Autodesk Inventor part; units mm, degrees
ref_plane "YZ Plane" through (0, 0, 0) normal (1, 0, 0) x (0, 1, 0)
ref_plane "XZ Plane" through (0, 0, 0) normal (0, 1, 0) x (-1, 0, 0)
ref_plane "XY Plane" through (0, 0, 0) normal (0, 0, 1) x (1, 0, 0)
sketch "Sketch1" plane through (0, 0, 0) normal (0, 0, 1) x (1, 0, 0)
  line L0 (0, 0) -> (25.4, 0)
  line L1 (25.4, 0) -> (25.4, -50.8)
  line L2 (25.4, -50.8) -> (0, -50.8)
  line L3 (0, -50.8) -> (0, 0)
  line L4 (22.225, -3.175) -> (3.175, -3.175)
  line L5 (3.175, -3.175) -> (3.175, -47.625)
  line L6 (3.175, -47.625) -> (22.225, -47.625)
  line L7 (22.225, -47.625) -> (22.225, -3.175)
  dimension "d0" = 25.4
  dimension "d1" = 50.8
  dimension "d2" = 3.175
extrude "Extrusion1" add sketch "Sketch1" along normal blind 127
sketch "Sketch2" plane through (0, 0, 0) normal (0, 1, 0) x (1, 0, 0)
  circle A0 centre (12.7, -12.7) radius 11.1125
  line L0 (0, 0) -> (0, -127)
  line L1 (0, 0) -> (25.4, 0)
  circle A1 centre (12.7, -112.0904) radius 11.1125
  circle A2 centre (12.7, -211.4809) radius 11.1125
  dimension "d5" = 12.7
  dimension "d6" = 12.7
  dimension "d7" = 22.225
  dimension "d8" = 99.3904
  dimension "d9" = 99.3904
  dimension "d10" = 12.7
  dimension "d11" = 22.225
  dimension "d12" = 12.7
  dimension "d13" = 22.225
extrude "Extrusion2" cut sketch "Sketch2" against normal blind 127
sketch "Sketch3" plane through (25.4, -50.8, 0) normal (1, 0, 0) x (0, 0, -1)
  line L0 (0, 44.45) -> (-63.5, 44.45)
  line L1 (-63.5, 44.45) -> (-63.5, 6.35)
  line L2 (-63.5, 6.35) -> (0, 6.35)
  line L3 (0, 6.35) -> (0, 44.45)
  line L4 (0, 50.8) -> (-127, 50.8)
  line L5 (0, 0) -> (-127, 0)
  line L6 (0, 50.8) -> (0, 0)
  dimension "d19" = 6.35
  dimension "d20" = 6.35
  dimension "d21" = 38.1
  dimension "d22" = 63.5
  dimension "d23" = 0
extrude "Extrusion3" cut sketch "Sketch3" against normal blind 127
properties part number "C Arm"
Verification items for the finished model (mm, model axes). A direction names the side the tool comes from. Round coordinates to 2 decimals unless told otherwise and drop trailing zeros. Write each loop counter-clockwise with the first axis right and the second up, starting at its lowest first coordinate (ties: lowest second). Pieces come first, ordered by that corner, then holes.
(1) Section check D-D (z = 12.7). Enter the section's corners in (x, y), plus the area to 3 significant figures.
Returned:
outline: (0, -50.8) - (1.59, -50.8) - (1.59, -44.45) - (0, -44.45) - close; (0, -6.35) - (1.59, -6.35) - (1.59, 0) - (0, 0) - close; (23.81, -50.8) - (25.4, -50.8) - (25.4, -44.45) - (23.81, -44.45) - close; (23.81, -6.35) - (25.4, -6.35) - (25.4, 0) - (23.81, 0) - close
area: 40.3 mm2
(2) Section check C-C (x = 12.7). Enter the section's corners in (y, z) (1 decimal).
Returned:
outline: (-50.8, 0) - (-47.6, 0) - (-47.6, 1.6) - (-50.8, 1.6) - close; (-50.8, 23.8) - (-47.6, 23.8) - (-47.6, 101) - (-50.8, 101) - close; (-50.8, 123.2) - (-47.6, 123.2) - (-47.6, 127) - (-50.8, 127) - close; (-3.2, 0) - (0, 0) - (0, 1.6) - (-3.2, 1.6) - close; (-3.2, 23.8) - (0, 23.8) - (0, 101) - (-3.2, 101) - close; (-3.2, 123.2) - (0, 123.2) - (0, 127) - (-3.2, 127) - close
(3) Material ranges on line 1 (Z direction, x = 12.7, y = -2.5); line 2 (Y direction, x = 15.5, z = 33) (3 decimals); line 3 (X direction, y = -46, z = 76) (3 decimals), recorded low to high.
Returned:
line 1: z = 0 to 1.59, 23.81 to 100.98, 123.2 to 127
line 2: y = -50.8 to -47.625, -3.175 to 0
line 3: x = 0 to 3.175, 22.225 to 25.4
(4) Mould release check, pull along X, two halves, no side actions. Record for faces 4 (the flat face through (25.4, -25, 91)), 5 (the flat face through (0, -26, 91)), 6 (the flat face through (3.175, -25, 122)): pulls with the +X half, pulls with the -X half, needs draft (parallel to the pull), parting line crosses it, or undercut.
Returned:
face 4: pulls with the +X half
face 5: pulls with the -X half
face 6: undercut
(5) Access from +Z, -Z, +X, -X, +Y, -Y to the whole of each face (thin tool, end or side, straight path). Record for faces 1 (the cylindrical face through (23.3, -2.42, 9.36)), 2 (the flat face through (24, -25, 63.5)), 3 (the flat face through (3.175, -25, 81)).
Returned:
face 1: +Y, -Y
face 2: -Z, +X, -X
face 3: +Z, -Z
(6) Section check B-B (y = -26). Enter the section's corners in (x, z) (1 decimal), plus the area to 3 significant figures.
Returned:
outline: (0, 63.5) - (3.2, 63.5) - (3.2, 106.4) arc R11.1 cw to (3.2, 117.8) - (3.2, 127) - (0, 127) - close; (22.2, 63.5) - (25.4, 63.5) - (25.4, 127) - (22.2, 127) - (22.2, 117.8) arc R11.1 cw to (22.2, 106.4) - close
area: 379 mm2
(7) Depth check by flat-ended pin: pin 1 Ø4 at (x, y) = (20, -12.5) entering from -Z; pin 2 Ø1.6 at (x, y) = (1.5, -30.5) entering from -Z. Enter the tip coordinate at first touch or a pass-through.
Returned:
pin 1: passes through
pin 2: stops at z = 63.5
(8) Section check A-A (z = 38). Enter the section's corners in (x, y) (3 decimals), plus the area to 3 significant figures.
Returned:
outline: (0, -50.8) - (25.4, -50.8) - (25.4, -44.45) - (22.225, -44.45) - (22.225, -47.625) - (3.175, -47.625) - (3.175, -44.45) - (0, -44.45) - close; (0, -6.35) - (3.175, -6.35) - (3.175, -3.175) - (22.225, -3.175) - (22.225, -6.35) - (25.4, -6.35) - (25.4, 0) - (0, 0) - close
area: 202 mm2
